Source: CAD feature listing. Evaluate the final solid. Frame: model axes, mm. A direction names the side the tool comes from. Coordinates: 2 decimals unless noted, no trailing zeros. Loops run counter-clockwise (first coordinate to the right, second up) from the corner with the lowest first, then second, coordinate; pieces in that order, holes last.
```python
from build123d import *

# Parameters (mm, degrees)
SKETCH1_R                = 2.5
BOSS_EXTRUDE1_DEPTH      = 2
BOSS_EXTRUDE2_DEPTH      = 2
BOSS_EXTRUDE3_DEPTH      = 18
BOSS_EXTRUDE3_DEPTH_BACK = 2
SKETCH4_W                = 31.798989874
SKETCH4_H                = 3.966560298
BOSS_EXTRUDE5_START      = -2
SKETCH6_R                = 2.5
BOSS_EXTRUDE5_DEPTH      = 2
FILLET1_R                = 10
FILLET2_R                = 10
FILLET4_R                = 4
CUT_EXTRUDE1_DEPTH       = 94.156093248


with BuildPart() as part:
    # Sketch1 → Boss-Extrude1 (new body)
    with BuildSketch(Plane(origin=(0, 0, 0), x_dir=(1, 0, 0), z_dir=(0, 1, 0))):
        with BuildLine():
            Line((0, 7), (25, 7))
            ThreePointArc((25, 7), (32, 0), (25, -7))
            Line((25, -7), (0, -7))
            ThreePointArc((0, -7), (-7, 0), (0, 7))
        make_face()
        with Locations(Location((0, 0, 0), (0, 0, 270))):
            Circle(SKETCH1_R, mode=Mode.SUBTRACT)
        with Locations(Location((25, 0, 0), (0, 0, 270))):
            Circle(SKETCH1_R, mode=Mode.SUBTRACT)
    extrude(amount=BOSS_EXTRUDE1_DEPTH)

    # Sketch3 → Boss-Extrude2 (add)
    with BuildSketch(Plane(origin=(0, 0, 0), x_dir=(-1, 0, 0), z_dir=(0, -1, 0))):
        with BuildLine():
            Line((-25, -7), (-36.715728753, -7))
            ThreePointArc((-36.715728753, -7), (-44.3693974, -8.52240935), (-50.857864376, -12.857864376))
            Line((-50.857864376, -12.857864376), (-61.970562748, -23.970562748))
            Line((-61.970562748, -23.970562748), (-81.769552622, -23.970562748))
            Line((-81.769552622, -23.970562748), (-71.870057685, -14.071067812))
            Line((-71.870057685, -14.071067812), (-56.656854249, 1.142135624))
            ThreePointArc((-56.656854249, 1.142135624), (-50.168387273, 5.47759065), (-42.514718626, 7))
            Line((-42.514718626, 7), (-25, 7))
            ThreePointArc((-25, 7), (-32, 0), (-25, -7))
        make_face()
    boss_extrude2 = extrude(amount=-BOSS_EXTRUDE2_DEPTH)

    # Sketch4 → Boss-Extrude3 (add, two sides: drawn at the far end of the back side and taken through both)
    with BuildSketch(Plane(origin=(0, 2, 0), x_dir=(1, 0, 0), z_dir=(0, 1, 0)).offset(-BOSS_EXTRUDE3_DEPTH_BACK)):
        with Locations((71.870057685, -21.987282599)):
            Rectangle(SKETCH4_W, SKETCH4_H)
    extrude(amount=BOSS_EXTRUDE3_DEPTH + BOSS_EXTRUDE3_DEPTH_BACK)

    # Mirror1: Boss-Extrude2 across plane
    add(boss_extrude2.mirror(Plane.ZX.offset(10)))

    # Sketch6 → Boss-Extrude5 (add)
    with BuildSketch(Plane(origin=(0, 20, 0), x_dir=(1, 0, 0), z_dir=(0, 1, 0)).offset(BOSS_EXTRUDE5_START)):
        with BuildLine():
            Line((25, -7), (0, -7))
            ThreePointArc((0, -7), (-7, 0), (0, 7))
            Line((0, 7), (25, 7))
            ThreePointArc((25, 7), (32, 0), (25, -7))
        make_face()
        with Locations(Location((0, 0, 0), (0, 0, 270))):
            Circle(SKETCH6_R, mode=Mode.SUBTRACT)
        with Locations(Location((25, 0, 0), (0, 0, 270))):
            Circle(SKETCH6_R, mode=Mode.SUBTRACT)
    extrude(amount=BOSS_EXTRUDE5_DEPTH)

    # Fillet1
    # the kernel refuses this fillet: 10 mm, written as the material it adds along each edge
    with BuildSketch(Plane(origin=(58.00400245, 0, 20.00400245), x_dir=(-1, 0, 0), z_dir=(0, 1, 0)), Plane(origin=(58.00400245, 18, 20.00400245), x_dir=(-1, 0, 0), z_dir=(0, 1, 0))) as fillet1_piece_1:
        with BuildLine():
            CenterArc((11.740850866, 2.401284758), FILLET1_R, 193.894123227, 31.105876773)
            Line((4.669783054, -4.669783054), (0, 0))
            Line((0, 0), (2.033439702, 0))
        make_face()
    extrude(amount=2)
    with BuildSketch(Plane(origin=(58.00400245, -16.510176322, 20.00400245), x_dir=(-1, 0, 0), z_dir=(0, 1, 0))) as fillet1_piece_2_section:
        with BuildLine():
            CenterArc((11.740850866, 2.401284758), FILLET1_R, 193.894123227, 31.105876773)
            Line((4.669783054, -4.669783054), (0, 0))
            Line((0, 0), (2.033439702, 0))
        make_face()
    fillet1_piece_2 = extrude(amount=35.020352644, mode=Mode.PRIVATE)
    fillet1_piece_2 = split(fillet1_piece_2, bisect_by=Plane(origin=(54.988670777, 18, 17.479262968), z_dir=(0, 1, 0)), keep=Keep.TOP, mode=Mode.PRIVATE)
    add(fillet1_piece_2)
    with BuildSketch(Plane(origin=(58.00400245, 1.489823678, 20.00400245), x_dir=(-1, 0, 0), z_dir=(0, 1, 0))) as fillet1_piece_3_section:
        with BuildLine():
            CenterArc((11.740850866, 2.401284758), FILLET1_R, 193.894123227, 31.105876773)
            Line((4.669783054, -4.669783054), (0, 0))
            Line((0, 0), (2.033439702, 0))
        make_face()
    fillet1_piece_3 = extrude(amount=35.020352644, mode=Mode.PRIVATE)
    fillet1_piece_3 = split(fillet1_piece_3, bisect_by=Plane(origin=(54.988670777, 2, 17.479262968), z_dir=(0, -1, 0)), keep=Keep.TOP, mode=Mode.PRIVATE)
    add(fillet1_piece_3)

    # Fillet2
    fillet2_edges = [part.edges().sort_by_distance(p)[0] for p in [
        (77.802992324, 1, 20.00400245),
        (77.802992324, 19, 20.00400245),
    ]]
    fillet(fillet2_edges, radius=FILLET2_R)

    # Fillet4
    # the kernel refuses this fillet: 4 mm, written as the material it takes off along each edge
    with BuildSketch(Plane(origin=(87.769552622, 30, 20.00400245), x_dir=(0, 0, 1), z_dir=(0, -1, 0))) as fillet4_piece_1:
        with BuildLine():
            CenterArc((FILLET4_R, FILLET4_R), FILLET4_R, 180, 90)
            Line((0, FILLET4_R), (0, 0))
            Line((0, 0), (FILLET4_R, 0))
        make_face()
    extrude(amount=40, mode=Mode.SUBTRACT)

    # Sketch8 → Cut-Extrude1 (cut, through all)
    with BuildSketch(Plane.XZ):
        with BuildLine():
            Line((0, 5), (25, 5))
            Line((25, 5), (37.544155877, 5))
            ThreePointArc((37.544155877, 5), (45.197824525, 6.52240935), (51.686291501, 10.857864376))
            Line((51.686291501, 10.857864376), (60.832429575, 20.00400245))
            Line((60.832429575, 20.00400245), (58.00400245, 20.00400245))
            Line((58.00400245, 20.00400245), (50.528510621, 12.697308088))
            ThreePointArc((50.528510621, 12.697308088), (44.096826604, 8.479014089), (36.548775141, 7))
            Line((36.548775141, 7), (0, 7))
            Line((0, 7), (0, 5))
        make_face()
    extrude(amount=-CUT_EXTRUDE1_DEPTH, mode=Mode.SUBTRACT)


solid = part.part
```
Q1. Material intervals for line 1 along Y through (x, z) = (48, 4.5); line 2 along X through (y, z) = (0.8, 0); line 3 along Z through (x, y) = (57, 11), sorted ascending.
Q2. Section query A-A on x = 34. Return the cut outline in (y, z).
Q3. Section query C-C on z = 0. Return the cut outline in (x, y), then the cut area to 3 significant figures.
Q4. First-contact query: pin 1 Ø6 at (x, y) = (72, 13.5) entering from -Z; pin 2 Ø8 at (x, z) = (0, 0) entering from +Y; pin 3 Ø1.5 at (x, z) = (50.5, 13) entering from +Y; pin 4 Ø3 at (y, z) = (11.5, 22.5) entering from -X. Flat tips, straight axial feed; report the tip coordinate or a pass-through.
Q5. Section query B-B on z = 15. Return the cut outline in (x, y), then the cut area to 3 significant figures.
Q6. Reachability of faces 1 (the flat face through (37, 2, 4)), 2 (the flat face through (56.2, 0.99, 15.37)), 3 (the cylindrical face through (55.246, 0.986, 18.011)) from +Z, -Z, +X, -X, +Y, -Y: full face, straight path, thin tool, end or side. Return the list, or none.
Q7. Draft query along Z for faces 4 (the flat face through (19, 19, 5)), 5 (the cylindrical face through (-2.44, 0.99, -0.54)), 6 (the flat face through (55.971, 10, 22)). Return one class per face: released by +Z, released by -Z, zero draft, split by the parting line, or undercut.
Q8. Section query D-D on y = 6.25. Return the cut outline in (x, z).
Resolved:
1. line 1: y = 0 to 2, 18 to 20
1. line 2: x = -7 to -2.5, 2.5 to 22.5, 27.5 to 57.8
1. line 3: z = 20 to 23.97
2. outline: (0, -7) - (2, -7) - (2, 5) - (0, 5) - close; (18, -7) - (20, -7) - (20, 5) - (18, 5) - close
3. outline: (-7, 0) - (-2.5, 0) - (-2.5, 2) - (-7, 2) - close; (-7, 18) - (-2.5, 18) - (-2.5, 20) - (-7, 20) - close; (2.5, 0) - (22.5, 0) - (22.5, 2) - (2.5, 2) - close; (2.5, 18) - (22.5, 18) - (22.5, 20) - (2.5, 20) - close; (27.5, 0) - (57.8, 0) - (57.8, 2) - (27.5, 2) - close; (27.5, 18) - (57.8, 18) - (57.8, 20) - (27.5, 20) - close
3. area: 219 mm2
4. pin 1: stops at z = 20
4. pin 2: stops at y = 20
4. pin 3: passes through
4. pin 4: stops at x = 55.97
5. outline: (55.83, 0) - (72.8, 0) - (72.8, 2) - (55.83, 2) - close; (55.83, 18) - (72.8, 18) - (72.8, 20) - (55.83, 20) - close
5. area: 67.9 mm2
6. face 1: -Z, +X, -X
6. face 2: +Y, -Y
6. face 3: +Z, -X, +Y, -Y
7. face 4: released by +Z
7. face 5: undercut
7. face 6: zero draft
8. outline: (55.97, 20) - (83.77, 20) arc R4 ccw to (87.77, 23.97) - (55.97, 23.97) - close
